For this review, take the finished solid that the model builds, in its own axes (mm). Face numbers are marked on the shaded views. A direction names the side the tool comes from. Give positions to 0.01 mm unless a question says otherwise; leave off trailing zeros. Write each loop counter-clockwise with the first axis right and the second up, starting at its lowest first coordinate (ties: lowest second). Pieces come first, ordered by that corner, then holes. Notation, with made-up numbers: M -29.75,80.5 L -21.75,80.5 A20 ccw -21.75,104.5 Z; hole C 86,34.25 d9. An arc over 180 degrees is marked long. One line per item, written item: value. Start each with the question number.
Item 1: Consider section D-D, the plane y = -4.75. Write out the cut boundary in (x, z).
Item 2: To check wall thickness, follow probe 1 along X at (y, z) = (0.75, -5.5); probe 2 along Y at (x, z) = (-27.95, 8.5); probe 3 along X at (y, z) = (1.25, -8.5). State the ranges of each line that lie inside material, in increasing order.
Item 3: Tool access review of the marked faces 1, 2 and 3: name each direction out of +Z, -Z, +X, -X, +Y, -Y from which nothing blocks a thin tool from reaching the whole face with its end or side.
Item 4: Consider section A-A, the plane y = 0. Write out the cut boundary in (x, z).
Item 5: Clearance check with flat-ended pins moving along their axes: pin 1 Ø4 at (y, z) = (4.5, -5.5) entering from +X; pin 2 Ø3 at (y, z) = (-3.5, 1.5) entering from +X; pin 3 Ø4 at (x, z) = (-61.5, 6) entering from +Y; pin 4 Ø12 at (y, z) = (6, 4.5) entering from +X. State where each tip first meets the part, or that it passes through.
Item 6: Consider section B-B, the plane z = 0. Write out the cut boundary in (x, y).
Item 7: Consider section C-C, the plane x = -40. Write out the cut boundary in (y, z).
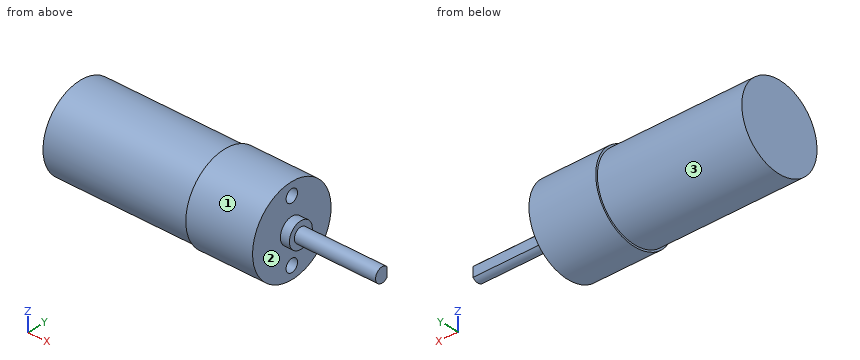
```python
from build123d import *

# Parameters (mm, degrees)
CUT_EXTRUDE1_START = -22.5
CUT_EXTRUDE1_DEPTH = 22.5
SKETCH4_R          = 1.75
CUT_EXTRUDE2_DEPTH = 5
SKETCH5_R          = 12
SKETCH5_R_2        = 11.5
CUT_EXTRUDE3_DEPTH = 40


with BuildPart() as part:
    # Sketch1 → Revolve1 (revolve)
    with BuildSketch(Plane(origin=(0, 0, 0), x_dir=(1, 0, 0), z_dir=(0, 1, 0)), mode=Mode.PRIVATE) as revolve1_sk:
        Polygon((-25, 12), (-83.5, 12), (-83.5, 0), (0, 0), (0, 2), (-22.5, 2), (-22.5, 3.5), (-25, 3.5), align=None)
    revolve(revolve1_sk.sketch.rotate(Axis((-83.5, 0, 0), (1, 0, 0)), 180), axis=Axis((-83.5, 0, 0), (1, 0, 0)))

    # Sketch2 → Cut-Extrude1 (cut)
    with BuildSketch(Plane(origin=(0, 0, 0), x_dir=(0, 0, -1), z_dir=(1, 0, 0)).offset(CUT_EXTRUDE1_START)):
        with BuildLine():
            Line((1.322875656, 1.5), (-1.322875656, 1.5))
            ThreePointArc((-1.322875656, 1.5), (0, 2), (1.322875656, 1.5))
        make_face()
    extrude(amount=CUT_EXTRUDE1_DEPTH, mode=Mode.SUBTRACT)

    # Sketch4 → Cut-Extrude2 (cut)
    with BuildSketch(Plane(origin=(-25, 0, 0), x_dir=(0, 0, -1), z_dir=(1, 0, 0))):
        with Locations((-8.5, 0)):
            Circle(SKETCH4_R)
        with Locations((8.5, 0)):
            Circle(SKETCH4_R)
    extrude(amount=-CUT_EXTRUDE2_DEPTH, mode=Mode.SUBTRACT)

    # Sketch5 → Cut-Extrude3 (cut)
    with BuildSketch(Plane.ZY.offset(83.5)):
        Circle(SKETCH5_R)
        Circle(SKETCH5_R_2, mode=Mode.SUBTRACT)
    extrude(amount=-CUT_EXTRUDE3_DEPTH, mode=Mode.SUBTRACT)


solid = part.part
```
Model answer:
1. outline: M -83.5,-10.47 L -43.5,-10.47 L -43.5,-11.02 L -25,-11.02 L -25,11.02 L -43.5,11.02 L -43.5,10.47 L -83.5,10.47 Z
2. probe 1: x = -83.5 to -25
2. probe 2: y = -8.47 to -1.75, 1.75 to 8.47
2. probe 3: x = -83.5 to -30
3. face 1: +X, -X
3. face 2: +X
3. face 3: -X
4. outline: M -83.5,-11.5 L -43.5,-11.5 L -43.5,-12 L -25,-12 L -25,-10.25 L -30,-10.25 L -30,-6.75 L -25,-6.75 L -25,-3.5 L -22.5,-3.5 L -22.5,-2 L 0,-2 L 0,2 L -22.5,2 L -22.5,3.5 L -25,3.5 L -25,6.75 L -30,6.75 L -30,10.25 L -25,10.25 L -25,12 L -43.5,12 L -43.5,11.5 L -83.5,11.5 Z
5. pin 1: stops at x = -25
5. pin 2: stops at x = -22.5
5. pin 3: stops at y = 10.78
5. pin 4: stops at x = 0
6. outline: M -83.5,-11.5 L -43.5,-11.5 L -43.5,-12 L -25,-12 L -25,-3.5 L -22.5,-3.5 L -22.5,-2 L 0,-2 L 0,1.5 L -22.5,1.5 L -22.5,3.5 L -25,3.5 L -25,12 L -43.5,12 L -43.5,11.5 L -83.5,11.5 Z
7. outline: C 0,0 d24
